Verification items for this drawing (mm, ordinates from the low corner). A direction names the side the tool comes from. Round coordinates to 2 decimals unless told otherwise and drop trailing zeros. Order: outer loops, then holes, each group sorted by start corner. A loop starts at its lowest first (then second) coordinate and runs counter-clockwise, first axis right, second up. Notation, with made-up numbers: M 58.25,85.5 L 65.25,85.5 A23 ccw 65.25,121.5 Z; hole C -4.5,25.25 d1. An arc over 180 degrees is marked long. Return JSON: item names as keys, results as strings. Group by question number.
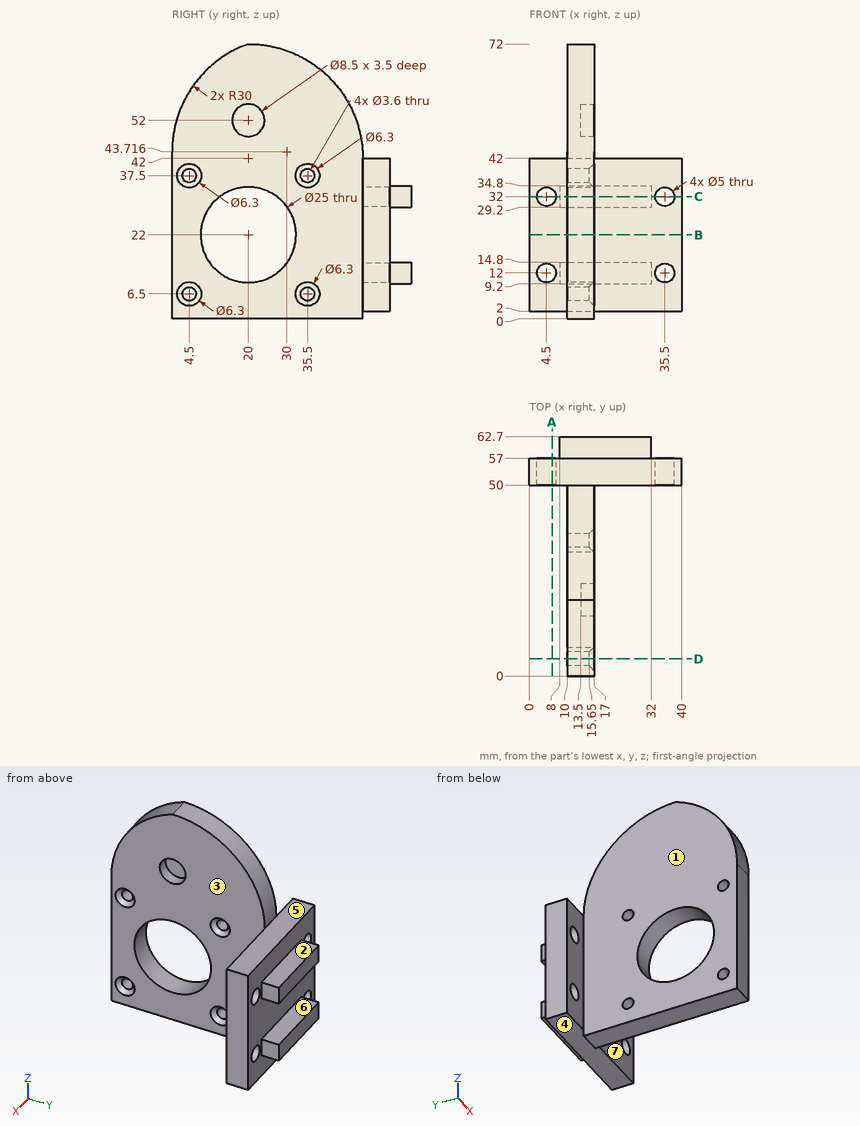
1. Thickness scan on line 1 along Y through (x, z) = (11.5, 37.5); line 2 along X through (y, z) = (54, 32); line 3 along Y through (x, z) = (12.5, 6). Record the ranges inside material, lowest first. Write a range as from..to.
2. Access from +Z, -Z, +X, -X, +Y, -Y to the whole of each face (thin tool, end or side, straight path). Record for the marked faces 1, 2 and 3.
3. Go/stop test with flat-tipped pins: pin 1 (12 mm diameter, centred on y = 10.5, z = 32, fed in from -X); pin 2 (4.5 mm diameter, centred on x = 17.5, y = 61, fed in from -Z); pin 3 (1.7 mm diameter, centred on y = 59, z = 33, fed in from +X). Record where each tip stops, or that it passes through.
4. Cross-section at A-A (x = 6). Enter the section's corners in (y, z), plus the area to 3 significant figures.
5. Cross-section at C-C (z = 32). Enter the section's corners in (x, y).
6. Draft check along Z on the marked faces 4, 5, 6 and 7. Enter one of: +Z half, -Z half, draft (parallel to the pull), parting line (faces both ways), or undercut.
7. Cross-section at B-B (z = 22). Enter the section's corners in (x, y).
8. Cross-section at D-D (y = 4.5). Enter the section's corners in (x, z).
Computed:
{
 "1": {"line 1": "y = 0..2.7, 6.3..33.7, 37.3..57", "line 2": "x = 0..2, 7..33, 38..40", "line 3": "y = 0..2.77, 6.23..33.77, 37.23..57"},
 "2": {"face 1": "+Z, -Z, -X, -Y", "face 2": "+Z, +X, -X, +Y", "face 3": "+Z, -Z, +X, -Y"},
 "3": {"pin 1": "stops at x = 10", "pin 2": "stops at z = 9.2", "pin 3": "stops at x = 32"},
 "4": {"outline": "M 50,2 L 57,2 L 57,10 L 50,10 Z; M 50,14 L 57,14 L 57,30 L 50,30 Z; M 50,34 L 57,34 L 57,42 L 50,42 Z", "area": "224 mm²"},
 "5": {"outline": "M 0,50 L 2,50 L 2,57 L 0,57 Z; M 7,50 L 10,50 L 10,27.5 L 17,27.5 L 17,50 L 33,50 L 33,57 L 32,57 L 32,62.7 L 8,62.7 L 8,57 L 7,57 Z; M 10,0 L 17,0 L 17,12.5 L 10,12.5 Z; M 38,50 L 40,50 L 40,57 L 38,57 Z"},
 "6": {"face 4": "-Z half", "face 5": "+Z half", "face 6": "undercut", "face 7": "draft"},
 "7": {"outline": "M 0,50 L 10,50 L 10,32.5 L 17,32.5 L 17,50 L 40,50 L 40,57 L 0,57 Z; M 10,0 L 17,0 L 17,7.5 L 10,7.5 Z"},
 "8": {"outline": "M 10,0 L 17,0 L 17,3.35 L 15.65,4.7 L 10,4.7 Z; M 10,8.3 L 15.65,8.3 L 17,9.65 L 17,34.35 L 15.65,35.7 L 10,35.7 Z; M 10,39.3 L 15.65,39.3 L 17,40.65 L 17,59.52 L 10,59.52 Z"}
}
